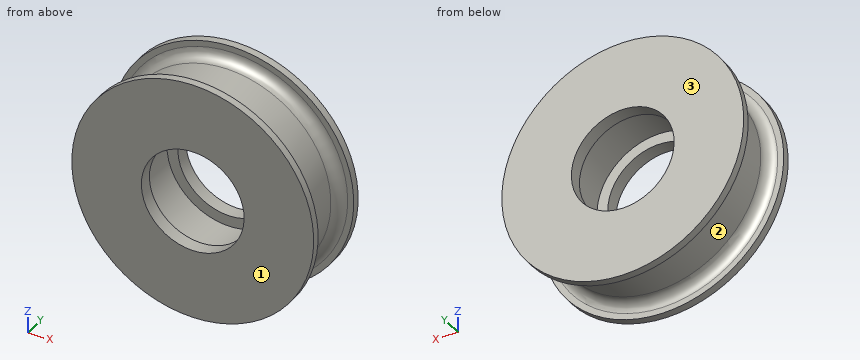
from build123d import *

# Parameters (mm, degrees)
SKETCH1_R           = 25.4
SKETCH1_R_2         = 13.081
BOSS_EXTRUDE1_DEPTH = 15.875
SKETCH7_R           = 15.875
SKETCH7_R_2         = 10.795
BOSS_EXTRUDE2_DEPTH = 2.8702
BOSS_EXTRUDE5_START = -2.8702
SKETCH9_R           = 15.875
SKETCH9_R_2         = 10.795
BOSS_EXTRUDE5_DEPTH = 2.8702


with BuildPart() as part:
    # Sketch1 → Boss-Extrude1 (new body)
    with BuildSketch(Plane(origin=(0, 0, 0), x_dir=(1, 0, 0), z_dir=(0, 1, 0))):
        with Locations(Location((0, 0, 0), (0, 0, 270))):
            Circle(SKETCH1_R)
        with Locations(Location((0, 0, 0), (0, 0, 270))):
            Circle(SKETCH1_R_2, mode=Mode.SUBTRACT)
    extrude(amount=BOSS_EXTRUDE1_DEPTH)

    # Sketch2 → Cut-Revolve1 (revolve, cut)
    with BuildSketch(Plane.XY, mode=Mode.PRIVATE) as cut_revolve1_sk:
        with BuildLine():
            Line((25.4, 14.2875), (24.13, 14.2875))
            ThreePointArc((24.13, 14.2875), (22.558455179, 13.636544821), (21.9075, 12.065))
            Line((21.9075, 12.065), (21.9075, 3.81))
            ThreePointArc((21.9075, 3.81), (22.558455179, 2.238455179), (24.13, 1.5875))
            Line((24.13, 1.5875), (25.4, 1.5875))
            Line((25.4, 1.5875), (25.4, 14.2875))
        make_face()
    revolve(cut_revolve1_sk.sketch.rotate(Axis((0, 0, 0), (0, 1, 0)), 90), axis=Axis((0, 0, 0), (0, 1, 0)), mode=Mode.SUBTRACT)

    # Sketch7 → Boss-Extrude2 (add)
    with BuildSketch(Plane.XZ):
        Circle(SKETCH7_R)
        with Locations(Location((0, 0, 0), (0, 0, 270))):
            Circle(SKETCH7_R_2, mode=Mode.SUBTRACT)
    extrude(amount=-BOSS_EXTRUDE2_DEPTH)

    # Sketch9 → Boss-Extrude5 (add)
    with BuildSketch(Plane(origin=(0, 15.875, 0), x_dir=(1, 0, 0), z_dir=(0, 1, 0)).offset(BOSS_EXTRUDE5_START)):
        Circle(SKETCH9_R)
        with Locations(Location((0, 0, 0), (0, 0, 90))):
            Circle(SKETCH9_R_2, mode=Mode.SUBTRACT)
    extrude(amount=BOSS_EXTRUDE5_DEPTH)


solid = part.part
Geometry: final body of the model. Coordinates: model frame, mm. Face numbers are marked on the shaded views. Round coordinates to 2 decimals unless told otherwise and drop trailing zeros. Order: outer loops, then holes, each group sorted by start corner. A loop starts at its lowest first (then second) coordinate and runs counter-clockwise, first axis right, second up. Notation, with made-up numbers: (-15.5, 68) - (33.5, 68) arc R19 cw to (33.5, 99) - close; hole circle Ø5 at (62, 46). An arc over 180 degrees is marked (long way). Write each question's results on one line, items separated by ' | '.
Item 1: Section A-A, the plane z = 0. Return the cut outline in (x, y) (1 decimal).
Completed:
outline: (-25.4, 0) - (-10.8, 0) - (-10.8, 2.9) - (-13.1, 2.9) - (-13.1, 13) - (-10.8, 13) - (-10.8, 15.9) - (-25.4, 15.9) - (-25.4, 14.3) - (-24.1, 14.3) arc R2.2 cw to (-21.9, 12.1) - (-21.9, 3.8) arc R2.2 cw to (-24.1, 1.6) - (-25.4, 1.6) - close; (10.8, 0) - (25.4, 0) - (25.4, 1.6) - (24.1, 1.6) arc R2.2 cw to (21.9, 3.8) - (21.9, 12.1) arc R2.2 cw to (24.1, 14.3) - (25.4, 14.3) - (25.4, 15.9) - (10.8, 15.9) - (10.8, 13) - (13.1, 13) - (13.1, 2.9) - (10.8, 2.9) - close
Item 2: Mould query, pull axis Y, two halves, no side actions, for the marked faces 1, 2 and 3. Classes: pulls with the +Y half, pulls with the -Y half, needs draft (parallel to the pull), parting line crosses it, or undercut.
Completed:
face 1: pulls with the -Y half | face 2: undercut | face 3: pulls with the +Y half
Item 3: First-contact query: pin 1 Ø8 at (x, y) = (-2, 10.5) entering from -Z; pin 2 Ø8 at (x, y) = (4, 9) entering from -Z; pin 3 Ø5 at (x, y) = (11.5, 12.5) entering from -Z; pin 4 Ø23.5 at (x, z) = (0, 0) entering from -Y. Flat tips, straight axial feed; report the tip coordinate or a pass-through.
Completed:
pin 1: z = -25.39 | pin 2: z = -21.91 | pin 3: z = -23.45 | pin 4: y = 0
Item 4: Section B-B, the plane x = 0. Return the cut outline in (y, z) (1 decimal), and give its area (3 significant figures).
Completed:
outline: (0, -25.4) - (1.6, -25.4) - (1.6, -24.1) arc R2.2 cw to (3.8, -21.9) - (12.1, -21.9) arc R2.2 cw to (14.3, -24.1) - (14.3, -25.4) - (15.9, -25.4) - (15.9, -10.8) - (13, -10.8) - (13, -13.1) - (2.9, -13.1) - (2.9, -10.8) - (0, -10.8) - close; (0, 10.8) - (2.9, 10.8) - (2.9, 13.1) - (13, 13.1) - (13, 10.8) - (15.9, 10.8) - (15.9, 25.4) - (14.3, 25.4) - (14.3, 24.1) arc R2.2 cw to (12.1, 21.9) - (3.8, 21.9) arc R2.2 cw to (1.6, 24.1) - (1.6, 25.4) - (0, 25.4) - close | area: 333 mm^2
Item 5: Material intervals for line 1 along Y through (x, z) = (-17, 17) (3 decimals); line 2 along Y through (x, z) = (-7.5, -10) (3 decimals); line 3 along X through (y, z) = (10.25, 0), sorted ascending. Write a range as [from, to].
Completed:
line 1: [0, 1.589], [14.286, 15.875] | line 2: [0, 2.87], [13.005, 15.875] | line 3: [-21.91, -13.08], [13.08, 21.91]
